Autodesk Inventor part; units mm, degrees
ref_plane "Work Plane1" through (0, 4, 0) normal (0, 1, 0) x (-1, 0, 0)
ref_plane "YZ Plane" through (0, 0, 0) normal (1, 0, 0) x (0, 1, 0)
ref_plane "XY Plane" through (0, 0, 0) normal (0, 0, 1) x (1, 0, 0)
sketch "Sketch1" plane through (0, 0, 0) normal (1, 0, 0) x (0, 1, 0)
  line L0 (0, 0) -> (4, 0)
  line L1 (4, 0) -> (4, -2)
  line L2 (4, -2) -> (6, -2)
  line L3 (6, -2) -> (6, -5)
  line L4 (6, -5) -> (0, -5)
  line L5 (0, -5) -> (0, 0)
  point P0 (3, -5)
  dimension "d0" = 5
  dimension "d1" = 2
  dimension "d2" = 8
  dimension "d3" = 12
revolve "Revolution1" add sketch "Sketch1" angle 360 about axis through (0, 0, -5) along (0, 0, 1)
sketch "Sketch2" plane through (0, 0, 0) normal (0, 0, 1) x (1, 0, 0)
  circle A0 centre (0, 0) radius 4
hole "Hole1" at (0, 0, 0) direction (0, 0, -1) diameter 6 depth 5
fillet "Fillet1" radius 0.85 1 edges at (0, -6, -5)
ref_plane "Work Plane1" through (0, 4, 0) normal (0, 1, 0) x (-1, 0, 0)
sketch "Sketch3" plane through (0, 4, 0) normal (0, 1, 0) x (-1, 0, 0)
  point P0 (0, 0)
  point P1 (0, -1)
  dimension "d14" = 1
hole "Hole2" at (0, 4, -1) direction (0, -1, 0) diameter 1 end through all
properties part number "03"
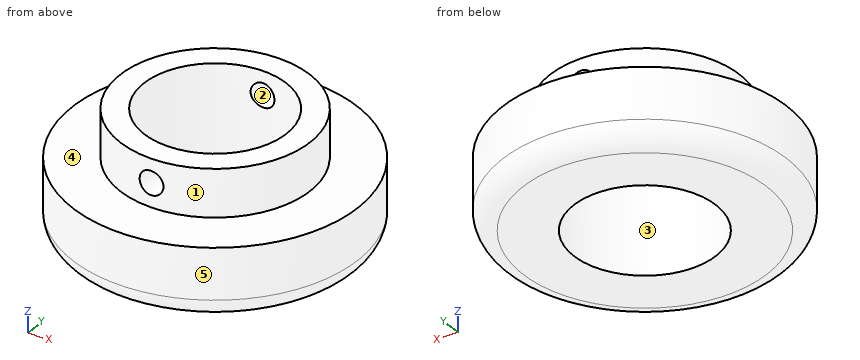
Design review of the part built by this model. Coordinates are the model's own, in mm. Face numbers are marked on the shaded views. A direction names the side the tool comes from. Coordinates: 2 decimals unless noted, no trailing zeros. Order: outer loops, then holes, each group sorted by start corner. A loop starts at its lowest first (then second) coordinate and runs counter-clockwise, first axis right, second up. Notation, with made-up numbers: M 7.5,9.25 L 46.5,9.25 A19 cw 46.5,24.25 Z; hole C 4,33.25 d3. An arc over 180 degrees is marked long. Use a Markdown table: item, result.
(1) Draft analysis for pull direction Y (two halves, no side actions). For the marked faces 3, 4 and 5, state which applies: released by +Y, released by -Y, zero draft, split by the parting line, or undercut.
Worked answers:
| item | result |
|---|---|
| face 3 | undercut |
| face 4 | zero draft |
| face 5 | split by the parting line |
(2) Add section B-B (x = 0). Give the boundary of the cut face in (y, z), then the cut area to 3 significant figures.
Worked answers:
| item | result |
|---|---|
| outline | M -6,-4.15 A0.85 ccw -5.15,-5 L -3,-5 L -3,-1.5 L -4,-1.5 L -4,-2 L -6,-2 Z; M -4,-0.5 L -3,-0.5 L -3,0 L -4,0 Z; M 3,-5 L 5.15,-5 A0.85 ccw 6,-4.15 L 6,-2 L 4,-2 L 4,-1.5 L 3,-1.5 Z; M 3,-0.5 L 4,-0.5 L 4,0 L 3,0 Z |
| area | 19.7 mm2 |
(3) Add section C-C (z = -0.7). Give the boundary of the cut face in (x, y).
Worked answers:
| item | result |
|---|---|
| outline | M -0.4,-3.98 L -0.4,-2.97 A3 cw -0.4,2.97 L -0.4,3.98 A4 ccw Z; M 0.4,-3.98 A4 ccw 0.4,3.98 L 0.4,2.97 A3 cw 0.4,-2.97 Z |
(4) For the marked faces 1 and 2, list the 3-axis set-ups (+Z, -Z, +X, -X, +Y, -Y) from which the entire face can be reached by the end or side of a thin tool; tool diameter is ignored.
Worked answers:
| item | result |
|---|---|
| face 1 | +Z |
| face 2 | +Y, -Y |
(5) For P1, Ø1, axis at x = 1, z = -2, coming from the +Y side; P2, Ø2, axis at y = -2, z = -4.5, coming from the +X side; P3, Ø2, axis at x = 3, z = -2.5, coming from the +Y side, all flat-tipped, find the tip position at first contact; note any pin that passes through.
Worked answers:
| item | result |
|---|---|
| P1 | stops at y = 5.98 |
| P2 | stops at x = 5.91 |
| P3 | stops at y = 5.66 |
(6) Add section A-A (y = 0). Give the boundary of the cut face in (x, z), then the cut area to 3 significant figures.
Worked answers:
| item | result |
|---|---|
| outline | M -6,-4.15 A0.85 ccw -5.15,-5 L -3,-5 L -3,0 L -4,0 L -4,-2 L -6,-2 Z; M 3,-5 L 5.15,-5 A0.85 ccw 6,-4.15 L 6,-2 L 4,-2 L 4,0 L 3,0 Z |
| area | 21.7 mm2 |
(7) Wall thickness on probe 1 along Z at (x, y) = (0, 3.4); probe 2 along Z at (x, y) = (3, 3.75); probe 3 along Y at (x, z) = (-1, -0.6): over which ranges is each line inside the solid? List them lowest first.
Worked answers:
| item | result |
|---|---|
| probe 1 | z = -5 to -1.5, -0.5 to 0 |
| probe 2 | z = -5 to -2 |
| probe 3 | y = -3.87 to -2.83, 2.83 to 3.87 |
